Answer from the drawing. Dimensions are ordinates in mm from the lowest x, y and z of the part. A direction names the side the tool comes from. Give positions to 0.01 mm unless a question says otherwise; leave off trailing zeros. Order: outer loops, then holes, each group sorted by start corner. A loop starts at its lowest first (then second) coordinate and runs counter-clockwise, first axis right, second up. Notation, with made-up numbers: (78, 49.5) - (110, 49.5) arc R15 cw to (110, 64.5) - close; hole circle Ø4 at (-26, 41.25). An arc over 180 degrees is marked (long way). Write each question's results on one line, items separated by ' | '.
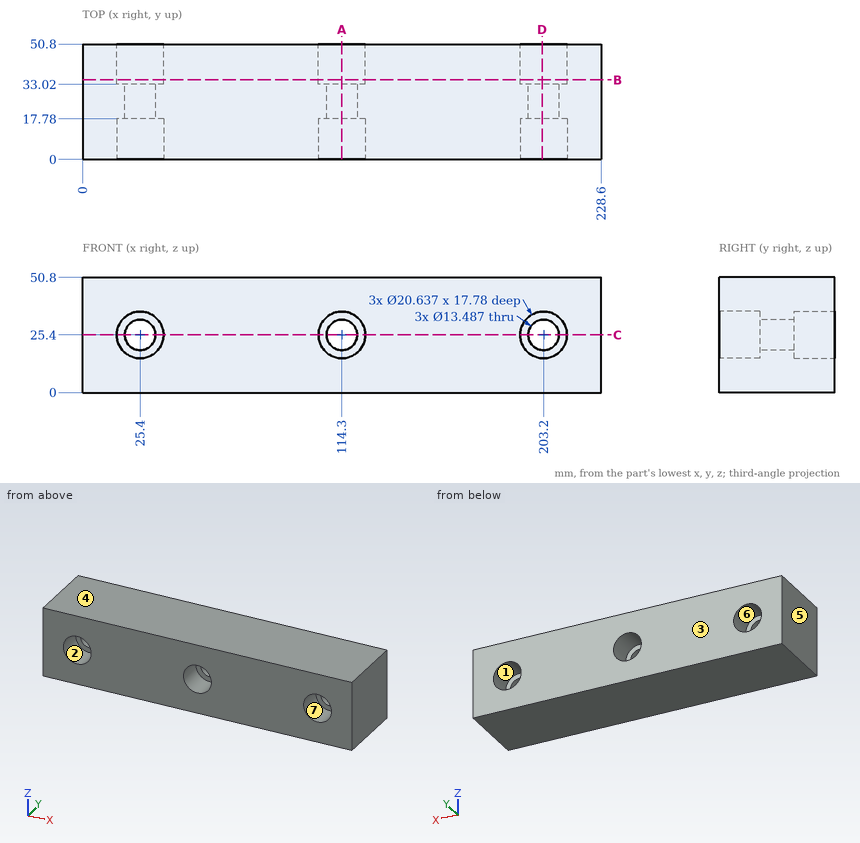
(1) Section C-C (z = 25.4) is taken. State how many separate pieces and enclosed holes the cut face has.
Conclusion:
separate pieces: 4 | enclosed holes: 0
(2) Section D-D (x = 202.5) is taken. Give the vertices of the cut face in (y, z) (1 decimal).
Conclusion:
outline: (0, 0) - (50.8, 0) - (50.8, 15.1) - (33, 15.1) - (33, 18.7) - (17.8, 18.7) - (17.8, 15.1) - (0, 15.1) - close; (0, 35.7) - (17.8, 35.7) - (17.8, 32.1) - (33, 32.1) - (33, 35.7) - (50.8, 35.7) - (50.8, 50.8) - (0, 50.8) - close
(3) Consider probe 1 along X at (y, z) = (14, 25); probe 2 along X at (y, z) = (28.5, 25.4); probe 3 along Z at (x, y) = (106.5, 33.5) (1 decimal). Determine where each line is inside the solid, lowest interval first. Write a range as [from, to].
Conclusion:
probe 1: [0, 15.09], [35.71, 103.99], [124.61, 192.89], [213.51, 228.6] | probe 2: [0, 18.66], [32.14, 107.56], [121.04, 196.46], [209.94, 228.6] | probe 3: [0, 18.6], [32.2, 50.8]
(4) Each of these flat-tipped pins is pushed along its axis until it touches: pin 1 (15.5 mm diameter, centred on x = 203.2, z = 25.4, fed in from -Y); pin 2 (8 mm diameter, centred on x = 114.3, z = 25.4, fed in from +Y). Where does it stop, or does it pass through?
Conclusion:
pin 1: y = 17.78 | pin 2: through
(5) For the marked faces 5, 6 and 7, determine the directions among +Z, -Z, +X, -X, +Y, -Y from which every point of the face is accessible in a straight line to the end or side of a thin tool.
Conclusion:
face 5: +Z, -Z, -X, +Y, -Y | face 6: +Y | face 7: -Y
(6) Section B-B (y = 35) is taken. Give the vertices of the cut face in (x, z), plus the area to 3 significant figures.
Conclusion:
outline: (0, 0) - (228.6, 0) - (228.6, 50.8) - (0, 50.8) - close; hole circle Ø20.64 at (25.4, 25.4); hole circle Ø20.64 at (114.3, 25.4); hole circle Ø20.64 at (203.2, 25.4) | area: 10,600 mm^2
(7) The mould has two halves that part along Z. Classify the marked faces 1, 2, 3 and 4: pulls with the +Z half, pulls with the -Z half, needs draft (parallel to the pull), parting line crosses it, or undercut.
Conclusion:
face 1: undercut | face 2: undercut | face 3: needs draft | face 4: pulls with the +Z half
(8) Section A-A (x = 114.3) is taken. Give the vertices of the cut face in (y, z).
Conclusion:
outline: (0, 0) - (50.8, 0) - (50.8, 15.08) - (33.02, 15.08) - (33.02, 18.66) - (17.78, 18.66) - (17.78, 15.08) - (0, 15.08) - close; (0, 35.72) - (17.78, 35.72) - (17.78, 32.14) - (33.02, 32.14) - (33.02, 35.72) - (50.8, 35.72) - (50.8, 50.8) - (0, 50.8) - close
